from build123d import *

# Parameters (mm, degrees)
SKETCH1_W           = 100
SKETCH1_H           = 100
SKETCH1_R           = 2.5
SKETCH1_W_2         = 3
SKETCH1_H_2         = 3
BOSS_EXTRUDE1_DEPTH = 5
SKETCH4_W           = 5
SKETCH4_H           = 10
BOSS_EXTRUDE2_DEPTH = 10
SKETCH5_R           = 2.5
CUT_EXTRUDE1_DEPTH  = 15


with BuildPart() as part:
    # Sketch1 → Boss-Extrude1 (new body)
    with BuildSketch(Plane(origin=(0, 0, 0), x_dir=(1, 0, 0), z_dir=(0, 1, 0))):
        Rectangle(SKETCH1_W, SKETCH1_H)
        with Locations((40, 40)):
            Circle(SKETCH1_R, mode=Mode.SUBTRACT)
        with Locations((-23.5, 23.5)):
            Rectangle(SKETCH1_W_2, SKETCH1_H_2, mode=Mode.SUBTRACT)
        with Locations((23.5, 23.5)):
            Rectangle(SKETCH1_W_2, SKETCH1_H_2, mode=Mode.SUBTRACT)
        with Locations((23.5, -23.5)):
            Rectangle(SKETCH1_W_2, SKETCH1_H_2, mode=Mode.SUBTRACT)
        with Locations((-23.5, -23.5)):
            Rectangle(SKETCH1_W_2, SKETCH1_H_2, mode=Mode.SUBTRACT)
        with Locations((4.5, 3)):
            Rectangle(SKETCH1_W_2, SKETCH1_H_2, mode=Mode.SUBTRACT)
        with Locations((-4.5, 3)):
            Rectangle(SKETCH1_W_2, SKETCH1_H_2, mode=Mode.SUBTRACT)
        with Locations((4.5, -3)):
            Rectangle(SKETCH1_W_2, SKETCH1_H_2, mode=Mode.SUBTRACT)
        with Locations((-4.5, -3)):
            Rectangle(SKETCH1_W_2, SKETCH1_H_2, mode=Mode.SUBTRACT)
    extrude(amount=BOSS_EXTRUDE1_DEPTH)

    # Sketch4 → Boss-Extrude2 (add)
    with BuildSketch(Plane(origin=(0, 5, 0), x_dir=(1, 0, 0), z_dir=(0, 1, 0))):
        with Locations((-42.5, -40)):
            Rectangle(SKETCH4_W, SKETCH4_H)
    extrude(amount=BOSS_EXTRUDE2_DEPTH)

    # Sketch5 → Cut-Extrude1 (cut)
    with BuildSketch(Plane.ZY.offset(45)):
        with Locations((40, 10)):
            Circle(SKETCH5_R)
    extrude(amount=-CUT_EXTRUDE1_DEPTH, mode=Mode.SUBTRACT)


solid = part.part
The model under review builds one solid part; all positions refer to its coordinate system, in mm. A direction names the side the tool comes from. Give positions to 0.01 mm unless a question says otherwise; leave off trailing zeros. Order: outer loops, then holes, each group sorted by start corner. A loop starts at its lowest first (then second) coordinate and runs counter-clockwise, first axis right, second up. Notation, with made-up numbers: M 42.25,25.25 L 48.25,25.25 A28 ccw 48.25,56.25 Z; hole C 33,17.25 d3. An arc over 180 degrees is marked long. One line per question, with ' | ' between items. Start each with the question number.
1) Clearance check with flat-ended pins moving along their axes: P1, Ø3, axis at x = 39, z = -30.5, coming from the +Y side; P2, Ø2.5, axis at x = -43.5, y = 11, coming from the +Z side; P3, Ø5.5, axis at x = -42, y = 11.5, coming from the -Z side. State where each tip first meets the part, or that it passes through.
2) Consider section A-A, the plane z = 40. Give the boundary of the cut face in (x, y).
3) Mouldability with a two-part tool opening along Z and no side actions: class faces 3 (the face through (-24, 2, 22)), 4 (the face through (-50, 2, 1)), 5 (the face through (-1, 2, -50)) as pulls with the +Z half, pulls with the -Z half, needs draft (parallel to the pull), parting line crosses it, or undercut.
4) Consider section D-D, the plane x = -16. Give the boundary of the cut face in (y, z).
5) Consider section C-C, the plane x = 40. Give the boundary of the cut face in (y, z).
6) Wall thickness on L1, parallel to X at y = 4.5, z = 23; L2, parallel to Y at x = -43.3, z = 40; L3, parallel to Z at x = 40, y = 2.6: over which ranges is each line inside the solid? List them lowest first. Write a range as from..to.
7) Consider section B-B, the plane y = 10. Give the boundary of the cut face in (x, z).
8) For faces 1 (the face through (-42.54, 9.04, 42.31)), 2 (the face through (4, 2, 4.5)), list the 3-axis set-ups (+Z, -Z, +X, -X, +Y, -Y) from which the entire face can be reached by the end or side of a thin tool; tool diameter is ignored.
Found:
1) P1: stops at y = 5 | P2: stops at z = 45 | P3: stops at z = 35
2) outline: M -50,0 L 50,0 L 50,5 L -40,5 L -40,7.5 L -45,7.5 L -45,5 L -50,5 Z; M -45,12.5 L -40,12.5 L -40,15 L -45,15 Z
3) face 3: undercut | face 4: needs draft | face 5: pulls with the -Z half
4) outline: M 0,-50 L 5,-50 L 5,50 L 0,50 Z
5) outline: M 0,-50 L 5,-50 L 5,-42.5 L 0,-42.5 Z; M 0,-37.5 L 5,-37.5 L 5,50 L 0,50 Z
6) L1: x = -50..-25, -22..22, 25..50 | L2: y = 0..7.5, 12.5..15 | L3: z = -50..-42.5, -37.5..50
7) outline: M -45,35 L -40,35 L -40,37.5 L -45,37.5 Z; M -45,42.5 L -40,42.5 L -40,45 L -45,45 Z
8) face 1: +X, -X | face 2: +Y, -Y
